Part print with two shaded views. Sizes in mm from the minimum x, y, z corner. A direction names the side the tool comes from. Coordinates: 2 decimals unless noted, no trailing zeros. Order: outer loops, then holes, each group sorted by start corner. A loop starts at its lowest first (then second) coordinate and runs counter-clockwise, first axis right, second up.
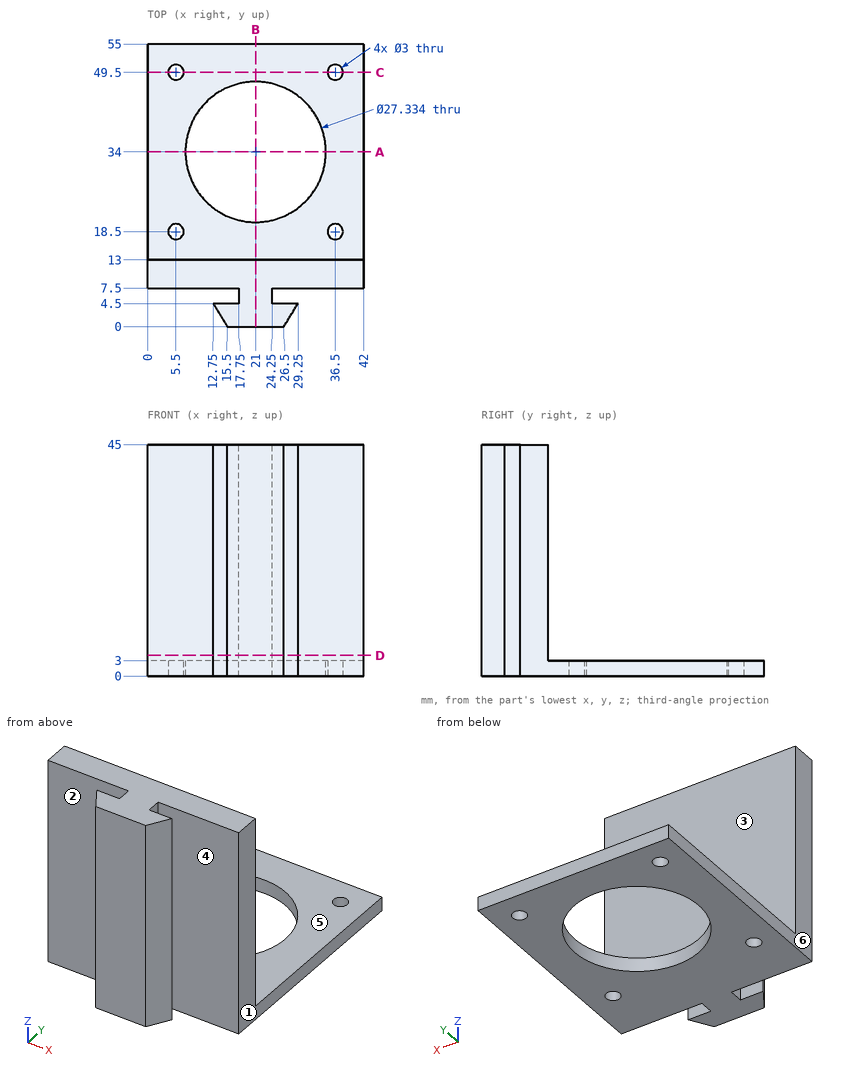
Q1. Wall check: line 1 along Y through (x, z) = (36.5, 0.8); line 2 along Y through (x, z) = (37, 28); line 3 along X through (y, z) = (5, 24.5). Give the ranges that are in metal, low to high.
Results list:
line 1: y = 7.5 to 17, 20 to 48, 51 to 55
line 2: y = 7.5 to 13
line 3: x = 17.75 to 24.25
Q2. Cut at D-D on z = 4. Write the cut outline in (x, y).
Results list:
outline: (0, 7.5) - (17.75, 7.5) - (17.75, 4.5) - (12.75, 4.5) - (15.5, 0) - (26.5, 0) - (29.25, 4.5) - (24.25, 4.5) - (24.25, 7.5) - (42, 7.5) - (42, 13) - (0, 13) - close
Q3. Mould opens along Y. For the marked faces 1, 2 and 3 say: pulls with the +Y half, pulls with the -Y half, needs draft (parallel to the pull), parting line crosses it, or undercut.
Results list:
face 1: needs draft
face 2: undercut
face 3: pulls with the +Y half
Q4. Cut at B-B on x = 21. Write the cut outline in (y, z), and give its area (3 significant figures).
Results list:
outline: (0, 0) - (20.33, 0) - (20.33, 3) - (13, 3) - (13, 45) - (0, 45) - close; (47.67, 0) - (55, 0) - (55, 3) - (47.67, 3) - close
area: 629 mm2
Q5. Which spindle directions (+Z, -Z, +X, -X, +Y, -Y) get a long thin tool onto all of the face, cutting with end or side? Do the marked faces 4, 5 and 6. Say none if no direction does.
Results list:
face 4: +Z, -Z, +X
face 5: +Z, +X, -X, +Y
face 6: +Z, -Z, -X, +Y, -Y
Q6. Cut at C-C on y = 49.5. Write the cut outline in (x, z), and give its area (3 significant figures).
Results list:
outline: (0, 0) - (4, 0) - (4, 3) - (0, 3) - close; (7, 0) - (35, 0) - (35, 3) - (7, 3) - close; (38, 0) - (42, 0) - (42, 3) - (38, 3) - close
area: 108 mm2
Q7. Pin check, flat tips, straight feed: pin 1 Ø1.5 at (x, z) = (26, 25.5) entering from +Y; pin 2 Ø6 at (x, y) = (31, 25) entering from +Z; pin 3 Ø1.8 at (x, y) = (5.5, 49.5) entering from +Z; pin 4 Ø5.5 at (x, z) = (35, 19) entering from -Y. Stop position of each tip, or through.
Results list:
pin 1: stops at y = 13
pin 2: stops at z = 3
pin 3: passes through
pin 4: stops at y = 7.5
Q8. Cut at A-A on y = 34. Write the cut outline in (x, z), and give its area (3 significant figures).
Results list:
outline: (0, 0) - (7.33, 0) - (7.33, 3) - (0, 3) - close; (34.67, 0) - (42, 0) - (42, 3) - (34.67, 3) - close
area: 44.0 mm2
